Build history of the part. All positions in model axes, mm. A direction names the side the tool comes from. Coordinates: 2 decimals unless noted, no trailing zeros. Order: outer loops, then holes, each group sorted by start corner. A loop starts at its lowest first (then second) coordinate and runs counter-clockwise, first axis right, second up. Notation, with made-up numbers: (16, -28.5) - (73, -28.5) arc R10 cw to (73, -19.5) - close; hole circle Ø6 at (56, -8). An arc over 180 degrees is marked (long way). Write each question's results on one line, items separated by ' | '.
Autodesk Inventor part; units mm, degrees
ref_plane "reduction" through (3, 0, 7) normal (-1, 0, 0) x (0, 0, 1)
ref_plane "YZ Plane" through (0, 0, 0) normal (1, 0, 0) x (0, 1, 0)
ref_plane "XZ Plane" through (0, 0, 0) normal (0, 1, 0) x (-1, 0, 0)
sketch "clawBase" plane through (0, 0, 0) normal (0, 1, 0) x (-1, 0, 0)
  line L0 (-3, -16.619) -> (0, -5)
  line L1 (0, -5) -> (0, 7)
  arc A0 (0, 7) -> (-3, -16.619) centre (0, -5) ccw
  arc A1 (0, 14) -> (-4.75, -23.3967) centre (0, -5) ccw
  line L2 (-3, -16.619) -> (-4.75, -23.3967)
  line L3 (0, 7) -> (0, 14)
  line L4 (0, 0) -> (0, 12)
  dimension "d3" = 12
  dimension "d5" = 7
  dimension "d6" = 0
  dimension "d7" = 5
  dimension "d8" = 3
  dimension "d11" = 12
  dimension "d12" = 0
extrude "clamp" add sketch "clawBase" against normal blind 10 contours L2 A1 L3 A0
ref_plane "reduction" through (3, 0, 7) normal (-1, 0, 0) x (0, 0, 1)
split "reductionSplit" plane through (3, 0, 7) removes the side toward (-1, 0, 0)
sketch "Sketch7" plane through (3, -10, 6.619) normal (-1, 0, 0) x (0, 0, 1)
  line L0 (0, 0) -> (0, 10)
  line L1 (7.1427, 0) -> (0, 0)
  line L2 (7.1427, 10) -> (7.1427, 0)
  line L3 (0, 10) -> (7.1427, 10)
  point P0 (-6.619, 10)
extrude "arm_c" add sketch "Sketch7" along normal blind 10
sketch "Sketch8" plane through (-7, 0, 13.7617) normal (0, 0, 1) x (1, 0, 0)
  line L0 (10, -10) -> (0, -10)
  line L1 (0, 0) -> (4, 0)
  line L2 (4, 0) -> (4, -10)
  line L3 (4, -10) -> (0, -10)
  line L4 (0, -10) -> (0, 0)
  point P0 (7, 0)
  dimension "d35" = 4
extrude "arb_b" add sketch "Sketch8" along normal blind 10
sketch "Sketch9" plane through (0, 0, 0) normal (0, 1, 0) x (1, 0, 0)
  line L0 (3, -6.619) -> (-7, -6.619)
  line L1 (3, -13.7617) -> (-3, -13.7617)
  point P0 (0, 0)
  point P1 (0, -10.1903)
  dimension "d39" = 7.1427
  dimension "d41" = 0
  dimension "d42" = 3.5714
hole "pinHole" at (0, 0, 10.1903) direction (0, -1, 0) diameter 3.25 end through all
sketch "Sketch10" plane through (3, -10, 6.619) normal (0, 0, -1) x (-1, 0, 0)
  line L0 (10, 10) -> (10, 0)
  line L1 (-3, 0) -> (10, 0)
  line L2 (10, 0) -> (10, 5.25)
  line L3 (10, 5.25) -> (-3, 5.25)
  line L4 (-3, 5.25) -> (-3, 0)
  line L5 (0, 10) -> (0, 0)
  line L6 (0, 0) -> (6, 0)
  point P0 (3, 10)
  point P1 (10, 0)
  dimension "d50" = 5.25
  dimension "d64" = 3
  dimension "d65" = 0
extrude "halfcut" cut sketch "Sketch10" along normal blind 4.25 and the other way blind 19.75
sketch "Sketch12" plane through (-7, -4.75, 6.619) normal (0, -1, 0) x (1, 0, 0)
  line L0 (0, 0) -> (0, 17.1427)
  line L1 (4, 7.1427) -> (4, 17.1427)
  line L2 (0, 17.1427) -> (4, 17.1427)
  line L3 (4, 17.1427) -> (4, 12.1427)
  line L4 (4, 12.1427) -> (0, 12.1427)
  line L5 (0, 12.1427) -> (0, 17.1427)
  line L6 (4, 7.1427) -> (10, 7.1427)
  point P0 (7, -6.619)
  point P1 (0, 12.1427)
  dimension "d68" = 5
extrude "Extrusion6" add sketch "Sketch12" along normal up to surface (5.25 mm away)
sketch "Sketch11" plane through (-3, 0, 23.7617) normal (1, 0, 0) x (0, 0, -1)
  line L0 (0, -10) -> (0, 0)
  line L1 (5, -10) -> (0, -10)
  point P0 (23.7617, 0)
  point P1 (2.5, -7.625)
  dimension "d71" = 2.5
  dimension "d72" = 2.375
hole "cableHole" at (-3, -7.625, 21.2617) direction (-1, 0, 0) diameter 2 end through all
equation "\"d3\" = r"
equation "\"d5\" = t"
equation "\"d8\" = 0.5 * a1"
equation "\"d11\" = r"
equation "\"d43\" = dpin"
equation "\"d57\" = dcable"
equation "\"r\" = 12"
equation "\"t\" = 7"
equation "\"a1\" = 6"
equation "\"fillet\" = 0.5"
equation "\"d14\" = -0.5 * a2"
equation "\"dpin\" = 3.25"
equation "\"tpinhole\" = t - dpin"
equation "\"linkb\" = d36 + 0.5 * t - d56"
equation "\"dcable\" = 2"
equation "\"a2\" = 6"
properties part number "holder2_base" material "Steel, Mild"
1. Tool access for faces 5 (the face through (-2, -4.75, 12)), 6 (the face through (6, -7, 9)), 7 (the face through (-2, -2, 6.619)), 8 (the face through (-5, -7, 18.762)), 9 (the face through (0, -2, 13.762)): list every direction of +Z, -Z, +X, -X, +Y, -Y with a clear straight run to the whole face (end or side of a thin tool).
Solved:
face 5: -X, -Y | face 6: +Z, -X, -Y | face 7: -Z, -X, +Y, -Y | face 8: -Z, +X, -X, -Y | face 9: +Z, +X, +Y, -Y
2. Band-saw the part on D-D on z = -10. Give the cut face in (x, y), then the cut area to 3 significant figures.
Solved:
outline: (10.91, -10) - (18.33, -10) - (18.33, 0) - (10.91, 0) - close | area: 74.2 mm2
3. Two-plate mould, pull along Y, no slides. Class faces 1 (the face through (-5, -10, 21)), 2 (the face through (-5, -8.3, 22)), 3 (the face through (10, 0, 4)), 4 (the face through (-3, -4, 20)): +Y half, -Y half, draft (parallel to the pull), parting line (faces both ways), or undercut.
Solved:
face 1: -Y half | face 2: undercut | face 3: +Y half | face 4: draft
4. Band-saw the part on A-A on x = 0. Give the cut face in (y, z).
Solved:
outline: (-4.75, 6.62) - (0, 6.62) - (0, 8.57) - (-4.75, 8.57) - close; (-4.75, 11.82) - (0, 11.82) - (0, 13.76) - (-4.75, 13.76) - close
5. Band-saw the part on C-C on x = 13. Give the cut face in (y, z), then the cut area to 3 significant figures.
Solved:
outline: (-10, -18.86) - (0, -18.86) - (0, 8.86) - (-10, 8.86) - close | area: 277 mm2
6. Drop flat-ended pins along their axis: pin 1 Ø4 at (y, z) = (-8, 10.5) entering from -X; pin 2 Ø4.5 at (x, y) = (-5.5, -6.5) entering from -Z; pin 3 Ø4 at (x, z) = (0, 10.19) entering from -Y. Give the stop position or say it passes through.
Solved:
pin 1: stops at x = 6 | pin 2: stops at z = 6.62 | pin 3: stops at y = -4.75
7. Probe line 1 (Z direction, x = 0, y = -3.35); line 2 (Z direction, x = 8.75, y = -5.25); line 3 (Z direction, x = -4.75, y = -2.5). List the from-to ranges inside material, lowest first.
Solved:
line 1: z = 6.62 to 8.57, 11.82 to 13.76 | line 2: z = -21.87 to -13.21, 3.21 to 11.87 | line 3: z = 6.62 to 23.76
